```python
from build123d import *

# Parameters (mm, degrees)
F1_DEPTH  = 2
F2_W      = 26
F2_H      = 26
F3_DEPTH  = 15.4
F4_W      = 35
F4_H      = 35
F4_W_2    = 37
F5_DEPTH  = 25
F6_W      = 26
F6_H      = 5
F7_DEPTH  = 25
F8_R      = 4
F9_R      = 2
F10_W     = 46
F10_H     = 46
F10_W_2   = 48
F11_DEPTH = 1
F12_R     = 1
F13_R     = 1
F0_W      = 6
F0_H      = 3
F0_W_2    = 3
F0_H_2    = 7
F14_DEPTH = 2


# Not quite as in the source:
# - a feature names something its author has since deleted; it is built from what else it names


with BuildPart() as f1:
    # F0 (on Top) → F1 (new body)
    with BuildSketch(Plane.XY):
        Polygon((173.5389735401, 18.1442317292), (-22.8906879723, 18.1442317292), (-22.8906879723, 13.5384923518), (-22.8906879723, 10.5384923518), (-22.8906879723, -31.8557682708), (-8.5117332786, -31.8557682708), (-5.5117332786, -31.8557682708), (187.1093120277, -31.8557682708), (187.1093120277, -31.4002893865), (187.1093120277, -28.4002893865), (187.1093120277, 18.1442317292), (176.5389735401, 18.1442317292), align=None)
    extrude(amount=F1_DEPTH)

    # F2 (on face) → F3 (cut)
    with BuildSketch(Plane(origin=(0, 0, 0), x_dir=(1, 0, 0), z_dir=(0, 0, -1))):
        with Locations((11.1093120277, 6.8557682708)):
            Rectangle(F2_W, F2_H)
    extrude(amount=-F3_DEPTH, mode=Mode.SUBTRACT)

    # F4 (on face) → F5 (cut)
    with BuildSketch(Plane(origin=(0, 0, 0), x_dir=(1, 0, 0), z_dir=(0, 0, -1))):
        with Locations((68.6093120277, 6.8557682708)):
            Rectangle(F4_W, F4_H)
        with Locations((153.6093120277, 6.8557682708)):
            Rectangle(F4_W_2, F4_H)
    extrude(amount=-F5_DEPTH, mode=Mode.SUBTRACT)

    # F6 (on face) → F7 (cut)
    with BuildSketch(Plane.XY.offset(2)):
        with Locations((11.1093120277, -29.3557682708)):
            Rectangle(F6_W, F6_H)
    extrude(amount=-F7_DEPTH, mode=Mode.SUBTRACT)

    # F8
    f8_edges = [f1.edges().sort_by_distance(p)[0] for p in [
        (-1.890688, -26.855768, 1),
        (24.109312, -26.855768, 1),
    ]]
    fillet(f8_edges, radius=F8_R)

    # F9
    f9_edges = [f1.edges().sort_by_distance(p)[0] for p in [
        (51.109312, 10.644232, 1),
        (86.109312, 10.644232, 1),
        (51.109312, -24.355768, 1),
        (135.109312, -24.355768, 1),
        (86.109312, -24.355768, 1),
        (172.109312, -24.355768, 1),
        (135.109312, 10.644232, 1),
        (172.109312, 10.644232, 1),
        (24.109312, 6.144232, 1),
        (-1.890688, 6.144232, 1),
        (24.109312, -19.855768, 1),
        (-1.890688, -19.855768, 1),
    ]]
    fillet(f9_edges, radius=F9_R)

    # F10 (on face) → F11 (cut)
    with BuildSketch(Plane.XY):
        with Locations((68.6093120277, -6.8557682708)):
            Rectangle(F10_W, F10_H)
        with Locations((153.6093120277, -6.8557682708)):
            Rectangle(F10_W_2, F10_H)
    extrude(amount=F11_DEPTH, mode=Mode.SUBTRACT)

    # F12
    f12_edges = [f1.edges().sort_by_distance(p)[0] for p in [
        (45.609312, -29.855768, 0.5),
        (91.609312, -29.855768, 0.5),
        (91.609312, 16.144232, 0.5),
        (45.609312, 16.144232, 0.5),
    ]]
    fillet(f12_edges, radius=F12_R)

    # F13
    f13_edges = [f1.edges().sort_by_distance(p)[0] for p in [
        (129.609312, -29.855768, 0.5),
        (177.609312, -29.855768, 0.5),
        (177.609312, 16.144232, 0.5),
        (129.609312, 16.144232, 0.5),
    ]]
    fillet(f13_edges, radius=F13_R)

    # F0 (on Top) → F14 (join)
    with BuildSketch(Plane.XY):
        with Locations((190.1093120277, -29.9002893865)):
            Rectangle(F0_W, F0_H)
        with Locations((175.0389735401, 21.6442317292)):
            Rectangle(F0_W_2, F0_H_2)
        with Locations((-7.0117332786, -35.3557682708)):
            Rectangle(F0_W_2, F0_H_2)
        with Locations((-25.8906879723, 12.0384923518)):
            Rectangle(F0_W, F0_H)
    extrude(amount=F14_DEPTH)


solid = f1.part
```
Read the model definition and answer for the solid it produces. Units are mm, in the model's axes. A direction names the side the tool comes from. Coordinates: 2 decimals unless noted, no trailing zeros. Write each loop counter-clockwise with the first axis right and the second up, starting at its lowest first coordinate (ties: lowest second). Pieces come first, ordered by that corner, then holes. Notation, with made-up numbers: (44, 5.25) -> (66, 5.25) arc R17 ccw to (66, 18.25) -> close; hole circle Ø10 at (89.25, 82). An arc over 180 degrees is marked (long way). Write item = value, one per line.
(1) Section A-A on y = 0.5 is taken. Write down the section's boundary in (x, z), plus the area to 3 significant figures.
From the geometry:
outline = (-22.89, 0) -> (-1.89, 0) -> (-1.89, 2) -> (-22.89, 2) -> close; (24.11, 0) -> (45.61, 0) -> (45.61, 1) -> (51.11, 1) -> (51.11, 2) -> (24.11, 2) -> close; (86.11, 1) -> (91.61, 1) -> (91.61, 0) -> (129.61, 0) -> (129.61, 1) -> (135.11, 1) -> (135.11, 2) -> (86.11, 2) -> close; (172.11, 1) -> (177.61, 1) -> (177.61, 0) -> (187.11, 0) -> (187.11, 2) -> (172.11, 2) -> close
area = 202 mm2
(2) Straight lines are drawn through the part: L1, parallel to X at y = 10.5, z = 0.6; L2, parallel to X at y = -10.5, z = 0.1; L3, parallel to X at y = 0.5, z = 1.3. For each, find the intervals that lie inside material, in ascending order. Write a range as from..to.
From the geometry:
L1 = -22.89..45.61, 91.61..129.61, 177.61..187.11
L2 = -22.89..-1.89, 24.11..45.61, 91.61..129.61, 177.61..187.11
L3 = -22.89..-1.89, 24.11..51.11, 86.11..135.11, 172.11..187.11
(3) Section D-D on x = 95.5 is taken. Write down the section's boundary in (y, z), plus the area to 3 significant figures.
From the geometry:
outline = (-31.86, 0) -> (18.14, 0) -> (18.14, 2) -> (-31.86, 2) -> close
area = 100 mm2
(4) Section B-B on x = 17 is taken. Write down the section's boundary in (y, z), plus the area to 3 significant figures.
From the geometry:
outline = (-26.86, 0) -> (-19.86, 0) -> (-19.86, 2) -> (-26.86, 2) -> close; (6.14, 0) -> (18.14, 0) -> (18.14, 2) -> (6.14, 2) -> close
area = 38.0 mm2
(5) Given pin 1 Ø0.8 at (x, z) = (159, 0.5) entering from -Y; pin 2 Ø14 at (x, y) = (145.5, -16.5) entering from -Z; pin 3 Ø0.5 at (y, z) = (-11.5, 0.5) entering from -X; pin 4 Ø0.8 at (x, z) = (159.5, 0.5) entering from +Y, each flat-ended and moving along its own axis, determine where each tip first touches the part or whether it passes through.
From the geometry:
pin_1 = -31.86
pin_2 = through
pin_3 = -22.89
pin_4 = 18.14
(6) For a pull along Y with two mould halves and no side action, classify faces 1 (the face through (81, 15, 2)), 2 (the face through (22.97, -28.06, 0.99)), 3 (the face through (153, -27, 1)) as +Y half, -Y half, draft (parallel to the pull), parting line (faces both ways), or undercut.
From the geometry:
face_1 = draft
face_2 = -Y half
face_3 = undercut
(7) Which of the six approach directions +Z, -Z, +X, -X, +Y, -Y give full straight-line access (tool end or side, diameter ignored) to faces 4 (the face through (89, -7, 1)), 5 (the face through (-0.75, -28.06, 0.99)), 6 (the face through (31, -6, 0))?
From the geometry:
face_4 = -Z
face_5 = +Z, -Z, -Y
face_6 = -Z, +X, -X, +Y, -Y
(8) Section C-C on z = 0.4 is taken. Count the separate pieces of the cut face and the enclosed holes in it, plus the area to 3 significant figures.
From the geometry:
separate_pieces = 1
enclosed_holes = 3
area = 5,460 mm2
